Geometry check sheet. Reference: the model listing, model coordinates, mm. Face numbers are marked on the shaded views. A direction names the side the tool comes from. Round coordinates to 2 decimals unless told otherwise and drop trailing zeros. Loops run counter-clockwise (first coordinate to the right, second up) from the corner with the lowest first, then second, coordinate; pieces in that order, holes last. Notation, with made-up numbers: (3, 7) -> (55, 7) arc R28 cw to (55, 33) -> close; hole circle Ø4 at (28.25, 48.25). An arc over 180 degrees is marked (long way). Use a Markdown table: item, result. Add a question column.
Q1. Material ranges on L1, parallel to Y at x = 0, z = -3.25; L2, parallel to Y at x = -12, z = -7.75; L3, parallel to X at y = -15.5, z = -8.5, recorded low to high.
Q2. Sectioned sample at C-C, the plane x = 13. Enter the section's corners in (y, z), then the cut area to 3 significant figures.
Q3. Sectioned sample at D-D, the plane z = -13. Enter the section's corners in (x, y).
Q4. Release check for a two-part mould opening along Y. For the marked faces 1, 2 and 3 record: released by +Y, released by -Y, zero draft, split by the parting line, or undercut.
Q5. Gauge pin test, flat ends, axial feed: P1, Ø3, axis at x = -24.18, y = 0, coming from the +Z side; P2, Ø1.5, axis at x = 16.5, z = -2.5, coming from the -Y side; P3, Ø7.5, axis at x = -14.5, z = -5.5, coming from the -Y side; P4, Ø1, axis at y = -17, z = -10, coming from the -X side. Record the tip position at first contact, or that the pin passes through.
Q6. Sectioned sample at A-A, the plane x = 0. Enter the section's corners in (y, z), then the cut area to 3 significant figures.
Q7. Sectioned sample at B-B, the plane y = -14. Enter the section's corners in (x, z).
Q8. Set-up check for the marked faces 4 and 5: record each of +Z, -Z, +X, -X, +Y, -Y from which the full face is reachable in a straight line by a thin tool's end or side.
```python
from build123d import *

# Parameters (mm, degrees)
SKETCH6_R                 = 29
SKETCH6_R_2               = 20
INNER_RING_DEPTH          = 15
MOTOR_CONNECTOR_CUT_DEPTH = 15
SKETCH8_R                 = 2.5
M3_HOLES_DEPTH            = 38
M3_HOLES_DEPTH_BACK       = 53
CUT_EXTRUDE1_DEPTH        = 16
CUT_EXTRUDE1_DEPTH_BACK   = 27


with BuildPart() as part:
    # Sketch6 → Inner Ring (new body)
    with BuildSketch(Plane.XY):
        Circle(SKETCH6_R)
        Circle(SKETCH6_R_2, mode=Mode.SUBTRACT)
    extrude(amount=-INNER_RING_DEPTH)

    # Sketch7 → Motor Connector Cut (add)
    with BuildSketch(Plane.XY):
        with BuildLine():
            ThreePointArc((20, 0), (19.840593925, 2.52008585), (19.364916731, 5))
            Line((19.364916731, 5), (9.999996731, 5))
            Line((9.999996731, 5), (9.999996731, -5))
            Line((9.999996731, -5), (19.364916731, -5))
            ThreePointArc((19.364916731, -5), (19.840593925, -2.52008585), (20, 0))
        make_face()
        with BuildLine():
            ThreePointArc((5, 19.364916731), (0, 20), (-5, 19.364916731))
            Line((-5, 19.364916731), (-5, 9.999996731))
            Line((-5, 9.999996731), (5, 9.999996731))
            Line((5, 9.999996731), (5, 19.364916731))
        make_face()
        with BuildLine():
            Line((-9.999996731, -5), (-9.999996731, 5))
            Line((-9.999996731, 5), (-19.364916731, 5))
            ThreePointArc((-19.364916731, 5), (-20, 0), (-19.364916731, -5))
            Line((-19.364916731, -5), (-9.999996731, -5))
        make_face()
        with BuildLine():
            Line((-5, -9.999996731), (-5, -19.364916731))
            ThreePointArc((-5, -19.364916731), (0, -20), (5, -19.364916731))
            Line((5, -19.364916731), (5, -9.999996731))
            Line((5, -9.999996731), (-5, -9.999996731))
        make_face()
    extrude(amount=-MOTOR_CONNECTOR_CUT_DEPTH)

    # Sketch8 → M3 Holes (cut, two sides)
    with BuildSketch(Plane.XY) as m3_holes_sk:
        with Locations((0, 24.182458366)):
            Circle(SKETCH8_R)
        with Locations((24.182458366, 0)):
            Circle(SKETCH8_R)
        with Locations((0, -24.182458366)):
            Circle(SKETCH8_R)
        with Locations((-24.182458366, 0)):
            Circle(SKETCH8_R)
    extrude(amount=M3_HOLES_DEPTH, mode=Mode.SUBTRACT)
    extrude(m3_holes_sk.sketch, amount=-M3_HOLES_DEPTH_BACK, mode=Mode.SUBTRACT)

    # Sketch9 → Cut-Extrude1 (cut, two sides)
    with BuildSketch(Plane(origin=(0, 0, -15), x_dir=(-1, 0, 0), z_dir=(0, 0, -1))) as cut_extrude1_sk:
        with BuildLine():
            Line((14.5, 25.11473671), (29, 0))
            ThreePointArc((29, 0), (25.11473671, 14.5), (14.5, 25.11473671))
        make_face()
        with BuildLine():
            Line((-29, 0), (-14.5, 25.11473671))
            ThreePointArc((-14.5, 25.11473671), (-25.11473671, 14.5), (-29, 0))
        make_face()
        with BuildLine():
            ThreePointArc((-29, 0), (-25.11473671, -14.5), (-14.5, -25.11473671))
            Line((-14.5, -25.11473671), (-29, 0))
        make_face()
        with BuildLine():
            ThreePointArc((14.5, -25.11473671), (25.11473671, -14.5), (29, 0))
            Line((29, 0), (14.5, -25.11473671))
        make_face()
    extrude(amount=CUT_EXTRUDE1_DEPTH, mode=Mode.SUBTRACT)
    extrude(cut_extrude1_sk.sketch, amount=-CUT_EXTRUDE1_DEPTH_BACK, mode=Mode.SUBTRACT)


solid = part.part
```
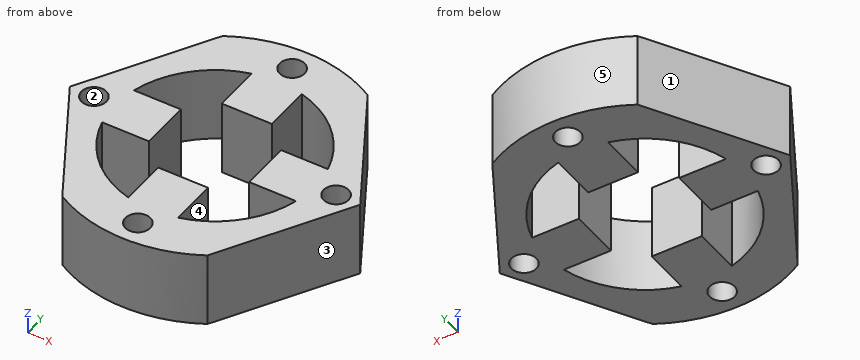
Values:
| question | item | result |
|---|---|---|
| 1 | L1 | -29 to -26.68, -21.68 to -10, 10 to 21.68, 26.68 to 29 |
| 1 | L2 | -26.4 to -16, -5 to 5, 16 to 26.4 |
| 1 | L3 | -20.05 to -12.64, -5 to 5, 12.64 to 20.05 |
| 2 | outline | (-25.92, -15) -> (-15.2, -15) -> (-15.2, 0) -> (-25.92, 0) -> close; (-5, -15) -> (5, -15) -> (5, 0) -> (-5, 0) -> close; (15.2, -15) -> (25.92, -15) -> (25.92, 0) -> (15.2, 0) -> close |
| 2 | area | 472 mm^2 |
| 3 | outline | (-29, 0) -> (-14.5, -25.11) arc R29 ccw to (14.5, -25.11) -> (29, 0) -> (14.5, 25.11) arc R29 ccw to (-14.5, 25.11) -> close; hole circle Ø5 at (-24.18, 0); hole (-19.36, -5) arc R20 ccw to (-5, -19.36) -> (-5, -10) -> (5, -10) -> (5, -19.36) arc R20 ccw to (19.36, -5) -> (10, -5) -> (10, 5) -> (19.36, 5) arc R20 ccw to (5, 19.36) -> (5, 10) -> (-5, 10) -> (-5, 19.36) arc R20 ccw to (-19.36, 5) -> (-10, 5) -> (-10, -5) -> close; hole circle Ø5 at (0, -24.18); hole circle Ø5 at (0, 24.18); hole circle Ø5 at (24.18, 0) |
| 4 | face 1 | released by +Y |
| 4 | face 2 | undercut |
| 4 | face 3 | released by -Y |
| 5 | P1 | through |
| 5 | P2 | y = -22.95 |
| 5 | P3 | y = -26.93 |
| 5 | P4 | x = -19.47 |
| 6 | outline | (-29, -15) -> (-26.68, -15) -> (-26.68, 0) -> (-29, 0) -> close; (-21.68, -15) -> (-10, -15) -> (-10, 0) -> (-21.68, 0) -> close; (10, -15) -> (21.68, -15) -> (21.68, 0) -> (10, 0) -> close; (26.68, -15) -> (29, -15) -> (29, 0) -> (26.68, 0) -> close |
| 6 | area | 420 mm^2 |
| 7 | outline | (-20.92, -15) -> (-14.28, -15) -> (-14.28, 0) -> (-20.92, 0) -> close; (-5, -15) -> (5, -15) -> (5, 0) -> (-5, 0) -> close; (14.28, -15) -> (20.92, -15) -> (20.92, 0) -> (14.28, 0) -> close |
| 8 | face 4 | +Z, -Z |
| 8 | face 5 | +Z, -Z, +Y |
